The model under review builds one solid part; all positions refer to its coordinate system, in mm. A direction names the side the tool comes from. Round coordinates to 2 decimals unless told otherwise and drop trailing zeros. Order: outer loops, then holes, each group sorted by start corner. A loop starts at its lowest first (then second) coordinate and runs counter-clockwise, first axis right, second up.
from build123d import *

# Parameters (mm, degrees)
SKETCH1_W           = 74
SKETCH1_H           = 21
BOSS_EXTRUDE1_DEPTH = 7.5
SKETCH2_R           = 8
CUT_EXTRUDE1_DEPTH  = 4.75
CUT_EXTRUDE1_TAPER  = -6
SKETCH4_R           = 2.6
CUT_EXTRUDE4_DEPTH  = 8.5000001
CHAMFER3_SIZE       = 5
CUT_EXTRUDE6_DEPTH  = 4
SKETCH11_R          = 2.25
CUT_EXTRUDE10_DEPTH = 8.5
FILLET4_R           = 1
FILLET5_R           = 1
CHAMFER5_SIZE       = 1
SKETCH12_R          = 8.1
SKETCH12_R_2        = 6.1
EXTRUDE_THIN1_DEPTH = 8.2
FILLET6_R           = 2
CHAMFER6_SIZE       = 1


with BuildPart() as part:
    # Sketch1 → Boss-Extrude1 (new body)
    with BuildSketch(Plane.XY):
        Rectangle(SKETCH1_W, SKETCH1_H)
    extrude(amount=BOSS_EXTRUDE1_DEPTH)

    # Sketch2 → Cut-Extrude1 (cut)
    with BuildSketch(Plane.XY.offset(7.5)):
        Circle(SKETCH2_R)
    extrude(amount=-CUT_EXTRUDE1_DEPTH, taper=CUT_EXTRUDE1_TAPER, mode=Mode.SUBTRACT)

    # Sketch4 → Cut-Extrude4 (cut, through all)
    with BuildSketch(Plane(origin=(0, 0, 0), x_dir=(-1, 0, 0), z_dir=(0, 0, -1))):
        with Locations((-25, 0)):
            Circle(SKETCH4_R)
        with Locations((25, 0)):
            Circle(SKETCH4_R)
    extrude(amount=-CUT_EXTRUDE4_DEPTH, mode=Mode.SUBTRACT)

    # Chamfer3
    chamfer3_edges = [part.edges().sort_by_distance(p)[0] for p in [
        (37, -10.5, 3.75),
        (-37, -10.5, 3.75),
        (-37, 10.5, 3.75),
        (37, 10.5, 3.75),
    ]]
    chamfer(chamfer3_edges, length=CHAMFER3_SIZE)

    # Sketch5 → Cut-Extrude6 (cut)
    with BuildSketch(Plane.XY.offset(7.5)):
        Polygon((22.690598923, -4), (27.309401077, -4), (29.618802154, 0), (27.309401077, 4), (22.690598923, 4), (20.381197846, 0), align=None)
        Polygon((-27.309401077, -4), (-22.690598923, -4), (-20.381197846, 0), (-22.690598923, 4), (-27.309401077, 4), (-29.618802154, 0), align=None)
    extrude(amount=-CUT_EXTRUDE6_DEPTH, mode=Mode.SUBTRACT)

    # Sketch11 → Cut-Extrude10 (cut, through all)
    with BuildSketch(Plane.XY.offset(7.5)):
        Circle(SKETCH11_R)
    extrude(amount=-CUT_EXTRUDE10_DEPTH, mode=Mode.SUBTRACT)

    # Fillet4
    fillet4_edges = [part.edges().sort_by_distance(p)[0] for p in [
        (27.6, 0, 0),
        (-22.4, 0, 0),
    ]]
    fillet(fillet4_edges, radius=FILLET4_R)

    # Fillet5
    fillet5_edges = [part.edges().sort_by_distance(p)[0] for p in [
        (-8, 0, 7.5),
    ]]
    fillet(fillet5_edges, radius=FILLET5_R)

    # Chamfer5
    chamfer5_edges = [part.edges().sort_by_distance(p)[0] for p in [
        (-37, 0, 0),
        (37, 0, 0),
        (0, -10.5, 0),
        (0, 10.5, 0),
    ]]
    chamfer(chamfer5_edges, length=CHAMFER5_SIZE)

    # Sketch12 → Extrude-Thin1 (add)
    with BuildSketch(Plane(origin=(0, 0, 0), x_dir=(-1, 0, 0), z_dir=(0, 0, -1))):
        Circle(SKETCH12_R)
        Circle(SKETCH12_R_2, mode=Mode.SUBTRACT)
    extrude(amount=EXTRUDE_THIN1_DEPTH)

    # Fillet6
    fillet6_edges = [part.edges().sort_by_distance(p)[0] for p in [
        (8.1, 0, 0),
    ]]
    fillet(fillet6_edges, radius=FILLET6_R)

    # Chamfer6
    chamfer6_edges = [part.edges().sort_by_distance(p)[0] for p in [
        (8.1, 0, -8.2),
    ]]
    chamfer(chamfer6_edges, length=CHAMFER6_SIZE)


solid = part.part
(1) The part is to be moulded in two halves that separate along Y. For faces 4 (the flat face through (-20, 0, 0)), 5 (the cylindrical face through (1.756, -7.907, -4.499)), 6 (the flat face through (-23, 2, 3.5)), say which applies: pulls with the +Y half, pulls with the -Y half, needs draft (parallel to the pull), parting line crosses it, or undercut.
(2) We need section B-B (x = -17). Give the boundary of the cut face in (y, z).
(3) To check wall thickness, follow L1, parallel to Y at x = 0, z = -2.25; L2, parallel to X at y = 1, z = 0.75; L3, parallel to Z at x = -19, y = 1.5. State the ranges of each line that lie inside material, in increasing order.
(4) Tool access review of faces 1 (the flat face through (-25, -4, 6)), 2 (the conical face through (7.845, 2.471, 5.357)), 3 (the cylindrical face through (-0.29, 2.23, 1.39)): name each direction out of +Z, -Z, +X, -X, +Y, -Y from which nothing blocks a thin tool from reaching the whole face with its end or side.
(5) Clearance check with flat-ended pins moving along their axes: P1, Ø6.5, axis at x = -25, y = 1, coming from the +Z side; P2, Ø6, axis at x = -2.5, y = -0.5, coming from the -Z side; P3, Ø3, axis at x = 25, y = 0, coming from the -Z side; P4, Ø1.5, axis at y = -6.5, z = 5.5, coming from the -X side. State where each tip first meets the part, or that it passes through.
(6) We need section A-A (x = -25). Give the boundary of the cut face in (y, z), and give its area (3 significant figures).
Verdict:
1. face 4: needs draft
1. face 5: parting line crosses it
1. face 6: undercut
2. outline: (-10.5, 1) - (-9.5, 0) - (9.5, 0) - (10.5, 1) - (10.5, 7.5) - (-10.5, 7.5) - close
3. L1: y = -8.1 to -6.1, 6.1 to 8.1
3. L2: x = -36.75 to -27.43, -22.57 to -2.02, 2.02 to 22.57, 27.43 to 36.75
3. L3: z = 0 to 7.5
4. face 1: +Z
4. face 2: none
4. face 3: +Z, -Z
5. P1: stops at z = 7.5
5. P2: stops at z = 0
5. P3: passes through
5. P4: stops at x = -36.75
6. outline: (-10.5, 1) - (-9.5, 0) - (-3.6, 0) arc R1 ccw to (-2.6, 1) - (-2.6, 3.5) - (-4, 3.5) - (-4, 7.5) - (-10.5, 7.5) - close; (2.6, 1) arc R1 ccw to (3.6, 0) - (9.5, 0) - (10.5, 1) - (10.5, 7.5) - (4, 7.5) - (4, 3.5) - (2.6, 3.5) - close
6. area: 106 mm2
